Part model, mm, in its own coordinate system. Give positions to 0.01 mm unless a question says otherwise; leave off trailing zeros. Order: outer loops, then holes, each group sorted by start corner. A loop starts at its lowest first (then second) coordinate and runs counter-clockwise, first axis right, second up. Notation, with made-up numbers: (-21.75, 70) - (16.25, 70) arc R13 ccw to (16.25, 82) - close; hole circle Ø1 at (13.5, 76). An arc over 180 degrees is marked (long way). Use a Markdown table: item, result. Add a question column.
from build123d import *

# Parameters (mm, degrees)
BOSS_EXTRUDE1_DEPTH = 1.5875
FILLET1_R           = 2.54
SKETCH2_R           = 2.2479
CUT_EXTRUDE1_DEPTH  = 2.5875


with BuildPart() as part:
    # Sketch1 → Boss-Extrude1 (new body)
    with BuildSketch(Plane(origin=(0, 0, 0), x_dir=(1, 0, 0), z_dir=(0, 1, 0))):
        Polygon((0, 0), (0, -48.432260883), (57.15, -48.432260883), (57.15, -33.090501198), (69.85, -33.090501198), (69.85, -12.7), (57.15, -12.7), (57.15, 0), align=None)
    extrude(amount=BOSS_EXTRUDE1_DEPTH)

    # Fillet1
    fillet1_edges = [part.edges().sort_by_distance(p)[0] for p in [
        (57.15, 0.79375, 0),
        (57.15, 0.79375, 12.7),
        (69.85, 0.79375, 12.7),
        (69.85, 0.79375, 33.090501198),
        (57.15, 0.79375, 33.090501198),
        (57.15, 0.79375, 48.432260883),
        (0, 0.79375, 48.432260883),
        (0, 0.79375, 0),
    ]]
    fillet(fillet1_edges, radius=FILLET1_R)

    # Sketch2 → Cut-Extrude1 (cut, through all)
    with BuildSketch(Plane(origin=(0, 1.5875, 0), x_dir=(1, 0, 0), z_dir=(0, 1, 0))):
        with Locations((3.175, -6.35)):
            Circle(SKETCH2_R)
        with Locations((3.175, -22.8854)):
            Circle(SKETCH2_R)
        with Locations((65.0748, -22.8854)):
            Circle(SKETCH2_R)
    extrude(amount=-CUT_EXTRUDE1_DEPTH, mode=Mode.SUBTRACT)


solid = part.part
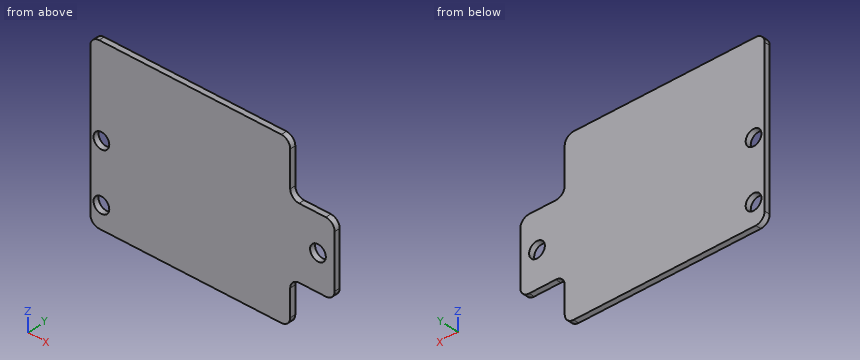
1. Cut at A-A (z = 6.35). Write the cut outline in (x, y), plus the area to 3 significant figures.
2. Cut at B-B (y = 1.2). State how many separate pieces and enclosed holes the cut face has, plus the area to 3 significant figures.
3. Pin check, flat tip, straight feed: P1, Ø4, axis at x = 65.07, z = 22.89, coming from the +Y side. Stop position of the tip, or through.
4. Drill centre lines: probe 1 along Z at (x, y) = (3, 0.7); probe 2 along X at (y, z) = (1.2, 6.35); probe 3 along X at (y, z) = (1.15, 41). Where is each one in solid material? Low to high. Write a range as [from, to].
Responses:
| question | item | result |
|---|---|---|
| 1 | outline | (0, 0) - (0.93, 0) - (0.93, 1.59) - (0, 1.59) - close; (5.42, 0) - (57.15, 0) - (57.15, 1.59) - (5.42, 1.59) - close |
| 1 | area | 83.6 mm² |
| 2 | separate pieces | 1 |
| 2 | enclosed holes | 3 |
| 2 | area | 2,970 mm² |
| 3 | P1 | passes through |
| 4 | probe 1 | z = [0, 4.11], [8.59, 20.64], [25.13, 48.43] |
| 4 | probe 2 | x = [0, 0.93], [5.42, 57.15] |
| 4 | probe 3 | x = [0, 57.15] |
